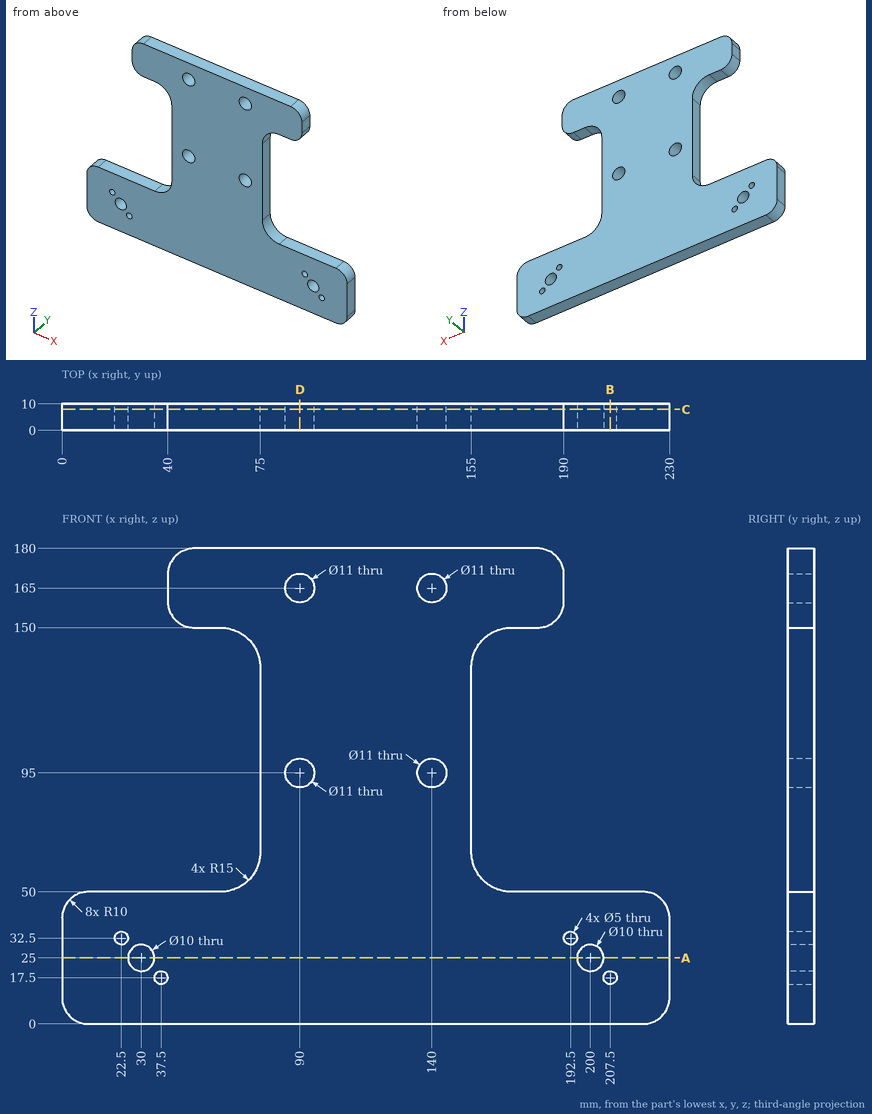
Print and shaded views of the part. All mm, measured from the part's lowest x, y and z. Give positions to 0.01 mm unless a question says otherwise; leave off trailing zeros. Loops run counter-clockwise (first coordinate to the right, second up) from the corner with the lowest first, then second, coordinate; pieces in that order, holes last. Notation, with made-up numbers: (57, -21) - (72, -21) arc R26 ccw to (72, 12) - close; hole circle Ø2 at (-14, -9.5). An arc over 180 degrees is marked (long way). One line per item, written item: value. Start each with the question number.
1. Slice it at A-A (z = 25). List the corners of the cut face in (x, y).
2. Slice it at C-C (y = 8). Give the number of separate pieces and of enclosed holes in the cut face, plus the area to 3 significant figures.
3. Pin check, flat tips, straight feed: pin 1 (5 mm diameter, centred on x = 26, y = 6, fed in from +Z); pin 2 (6.5 mm diameter, centred on x = 90, z = 165, fed in from +Y); pin 3 (5 mm diameter, centred on x = 186, y = 4.5, fed in from +Z); pin 4 (3 mm diameter, centred on y = 5.5, z = 95, fed in from +X). Stop position of each tip, or through.
4. Slice it at D-D (x = 90). List the corners of the cut face in (y, z).
5. Slice it at B-B (x = 207.5). List the corners of the cut face in (y, z), plus the area to 3 significant figures.
6. Probe L1, parallel to X at y = 5, z = 25; L2, parallel to Z at x = 140, y = 6.75; L3, parallel to Z at x = 200, y = 6. List the from-to ranges inside material, lowest first. Write a range as from..to.
Solution:
1. outline: (0, 0) - (25, 0) - (25, 10) - (0, 10) - close; (35, 0) - (195, 0) - (195, 10) - (35, 10) - close; (205, 0) - (230, 0) - (230, 10) - (205, 10) - close
2. separate pieces: 1
2. enclosed holes: 10
2. area: 23,400 mm^2
3. pin 1: stops at z = 50
3. pin 2: passes through
3. pin 3: stops at z = 179.37
3. pin 4: stops at x = 155
4. outline: (0, 0) - (10, 0) - (10, 89.5) - (0, 89.5) - close; (0, 100.5) - (10, 100.5) - (10, 159.5) - (0, 159.5) - close; (0, 170.5) - (10, 170.5) - (10, 180) - (0, 180) - close
5. outline: (0, 0) - (10, 0) - (10, 15) - (0, 15) - close; (0, 20) - (10, 20) - (10, 50) - (0, 50) - close
5. area: 450 mm^2
6. L1: x = 0..25, 35..195, 205..230
6. L2: z = 0..89.5, 100.5..159.5, 170.5..180
6. L3: z = 0..20, 30..50
